Check sheet for the modelled part. Datum: model origin and axes. Units: mm. A direction names the side the tool comes from. Round coordinates to 2 decimals unless told otherwise and drop trailing zeros. Write each loop counter-clockwise with the first axis right and the second up, starting at its lowest first coordinate (ties: lowest second). Pieces come first, ordered by that corner, then holes. Notation, with made-up numbers: (19.5, 27.25) - (62.5, 27.25) arc R17 cw to (62.5, 52.25) - close; hole circle Ø2 at (-16, 7). An arc over 180 degrees is marked (long way). Use one line per item in the form item = value. Start each with the question number.
1) Gauge pin test, flat ends, axial feed: P1, Ø6, axis at x = 2.5, z = 6.5, coming from the -Y side; P2, Ø1, axis at x = -4, y = 3, coming from the +Z side; P3, Ø1.5, axis at y = 2, z = 2, coming from the -X side. Record the tip position at first contact, or that the pin passes through.
2) Set-up check for faces 1 (the face through (3.3, 0.1, 0)), 2 (the face through (0, 0, 11)), 3 (the face through (0, 0, -4)): record each of +Z, -Z, +X, -X, +Y, -Y from which the full face is reachable in a straight line by a thin tool's end or side.
3) Section check A-A (y = 0). Record the boundary of the cut face in (x, z), then the cut area to 4 significant figures.
4) Section check C-C (z = -4.5). Record the boundary of the cut face in (x, y).
5) Section check D-D (z = 2.25). Record the boundary of the cut face in (x, y).
6) Scan lines: probe 1 along Y at (x, z) = (0, -10.5); probe 2 along Z at (x, y) = (0.5, 0.5); probe 3 along X at (y, z) = (1, -7.75). Record each from-to range of solid material in increasing order.
7) Draft check along Y on faces 4 (the face through (-1.08, -4.88, -6.41)), 5 (the face through (-2.579, 1.978, -8.563)), 6 (the face through (3.3, -1, -13)). Enter one of: +Y half, -Y half, draft (parallel to the pull), parting line (faces both ways), or undercut.
Autodesk Fusion 360 part; units mm, degrees
sketch "Sketch1" plane through (0, 0, 0) normal (0, 0, 1) x (1, 0, 0)
  circle A0 centre (0, 0) radius 3
  circle A1 centre (0, 0) radius 5
  dimension "d1" = 6
  dimension "d4" = 10
extrude "Extrude1" add sketch "Sketch1" along normal blind 11 contours A0
extrude "Extrude2" add sketch "Sketch1" against normal blind 13 contours A0 | A1
ref_plane "WorkPlane1" through (0, 0, -15) normal (0, 0, 1) x (1, 0, 0)
sketch "Sketch2" plane through (0, 0, -15) normal (0, 0, 1) x (1, 0, 0)
  circle A0 centre (0, 0) radius 3.25
  dimension "d8" = 6.5
extrude "Extrude3" cut sketch "Sketch2" along normal blind 11
Results are:
q1.P1 = -3
q1.P2 = 0
q1.P3 = -2.73
q2.face_1 = +Z
q2.face_2 = +Z, +X, -X, +Y, -Y
q2.face_3 = -Z
q3.outline = (-5, -13) - (-3.25, -13) - (-3.25, -4) - (3.25, -4) - (3.25, -13) - (5, -13) - (5, 0) - (3, 0) - (3, 11) - (-3, 11) - (-3, 0) - (-5, 0) - close
q3.area = 137.5 mm²
q4.outline = circle Ø10 at (0, 0); hole circle Ø6.5 at (0, 0)
q5.outline = circle Ø6 at (0, 0)
q6.probe_1 = -5 to -3.25, 3.25 to 5
q6.probe_2 = -4 to 11
q6.probe_3 = -4.9 to -3.09, 3.09 to 4.9
q7.face_4 = parting line
q7.face_5 = undercut
q7.face_6 = draft
